Model file for the job. Use its own axes, mm. Face numbers are marked on the shaded views. Coordinates: 2 decimals unless noted, no trailing zeros. Order: outer loops, then holes, each group sorted by start corner. A loop starts at its lowest first (then second) coordinate and runs counter-clockwise, first axis right, second up. Notation, with made-up numbers: (-31.75, 49) -> (-9.75, 49) arc R24 cw to (-9.75, 65) -> close; hole circle Ø10 at (68.25, -12.75). An arc over 180 degrees is marked (long way). Write item = value, one per line. Start each with the question number.
Q1. Flat gauge pins, fed straight in: pin 1 (3 mm diameter, centred on x = 2.5, y = 112, fed in from +Z); pin 2 (7 mm diameter, centred on y = 99.36, z = 75.68, fed in from -X); pin 3 (4 mm diameter, centred on x = -19.05, z = -9.525, fed in from +Y); pin 4 (8 mm diameter, centred on x = -8, z = 86.5, fed in from +Y). Where does each tip first touch, or does it go through?
Q2. Cut at B-B, the plane y = 158.75. List the corners of the cut face in (x, z) (3 decimals), plus the area to 3 significant figures.
Q3. Cut at A-A, the plane x = -5. List the corners of the cut face in (y, z) (3 decimals).
Q4. Cut at D-D, the plane x = -23.5. List the corners of the cut face in (y, z) (3 decimals).
Q5. Cut at C-C, the plane y = 39. List the corners of the cut face in (x, z) (3 decimals).
Q6. Wall check: line 1 (Z direction, x = -19, y = 4) (3 decimals); line 2 (Y direction, x = -15.5, z = 73). Give the ranges that are in metal, low to high. Write a range as from..to.
Q7. Mould opens along Y. For the marked faces 1, 2 and 3 say: +Y half, -Y half, draft (parallel to the pull), parting line (faces both ways), or undercut.
from build123d import *

# Parameters (mm, degrees)
BOSS_EXTRUDE1_DEPTH  = 6.35
SKETCH5_W            = 184.15
SKETCH5_H            = 6.35
BOSS_EXTRUDE4_DEPTH  = 31.75
SKETCH6_W            = 12.7
SKETCH6_H            = 88.9
CUT_EXTRUDE2_DEPTH   = 270.576010849
CUT_EXTRUDE3_REACH   = 277.64
SKETCH7_R            = 2.25
SKETCH7_W            = 59.436
SKETCH7_H            = 28.313784743
SKETCH8_R            = 6.35
CUT_EXTRUDE4_DEPTH   = 276.640473489
FILLET1_R            = 2.54
CONVERT_SOLID1_START = -34.925
CONVERT_SOLID1_DEPTH = 184.15
CUT_EXTRUDE5_REACH   = 277.64
CUT_EXTRUDE6_REACH   = 271.576
SKETCH10_R           = 1.63195


# Read off the part's stored shape, not the designer's step: Convert-Solid1
with BuildPart() as part:
    # Sketch1 → Boss-Extrude1 (new body)
    with BuildSketch(Plane(origin=(0, 0, 0), x_dir=(0, 0, -1), z_dir=(1, 0, 0))):
        with BuildLine():
            Line((-117.475, 228.6), (34.925, 228.6))
            Line((34.925, 228.6), (34.925, 8.89))
            Line((34.925, 8.89), (34.925, 0))
            Line((34.925, 0), (-34.925, 0))
            Line((-34.925, 0), (-34.925, 8.89))
            ThreePointArc((-34.925, 8.89), (-79.375, 53.34), (-123.825, 8.89))
            Line((-123.825, 8.89), (-123.825, 0))
            Line((-123.825, 0), (-149.225, 0))
            Line((-149.225, 0), (-149.225, 76.2))
            Line((-149.225, 76.2), (-117.475, 228.6))
        make_face()
    extrude(amount=BOSS_EXTRUDE1_DEPTH)

    # Sketch5 → Boss-Extrude4 (add)
    with BuildSketch(Plane.ZY):
        with Locations((57.15, 3.175)):
            Rectangle(SKETCH5_W, SKETCH5_H)
    extrude(amount=BOSS_EXTRUDE4_DEPTH)

    # Sketch6 → Cut-Extrude2 (cut, through all)
    with BuildSketch(Plane(origin=(0, 6.35, 0), x_dir=(1, 0, 0), z_dir=(0, 1, 0))):
        with Locations((-6.35, -79.375)):
            Rectangle(SKETCH6_W, SKETCH6_H)
    extrude(amount=-CUT_EXTRUDE2_DEPTH, mode=Mode.SUBTRACT)

    # Sketch7 → Cut-Extrude3 (cut, up to next)
    with BuildSketch(Plane(origin=(6.35, 0, 0), x_dir=(0, 0, -1), z_dir=(1, 0, 0)), mode=Mode.PRIVATE) as cut_extrude3_sk1:
        with Locations((-75.679460058, 116.337237118)):
            Circle(SKETCH7_R)
    cut_extrude3_tool1 = extrude(cut_extrude3_sk1.sketch, amount=-CUT_EXTRUDE3_REACH, mode=Mode.PRIVATE) & part.part
    # Sketch7 → Cut-Extrude3 (cut, up to next)
    with BuildSketch(Plane(origin=(6.35, 0, 0), x_dir=(0, 0, -1), z_dir=(1, 0, 0)), mode=Mode.PRIVATE) as cut_extrude3_sk2:
        with Locations((-75.679460058, 99.360389657)):
            Circle(SKETCH7_R)
    cut_extrude3_tool2 = extrude(cut_extrude3_sk2.sketch, amount=-CUT_EXTRUDE3_REACH, mode=Mode.PRIVATE) & part.part
    # Sketch7 → Cut-Extrude3 (cut, up to next)
    with BuildSketch(Plane(origin=(6.35, 0, 0), x_dir=(0, 0, -1), z_dir=(1, 0, 0)), mode=Mode.PRIVATE) as cut_extrude3_sk3:
        with Locations((-6.03755368, 99.360389657)):
            Circle(SKETCH7_R)
    cut_extrude3_tool3 = extrude(cut_extrude3_sk3.sketch, amount=-CUT_EXTRUDE3_REACH, mode=Mode.PRIVATE) & part.part
    # Sketch7 → Cut-Extrude3 (cut, up to next)
    with BuildSketch(Plane(origin=(6.35, 0, 0), x_dir=(0, 0, -1), z_dir=(1, 0, 0)), mode=Mode.PRIVATE) as cut_extrude3_sk4:
        with Locations((-6.03755368, 116.337237118)):
            Circle(SKETCH7_R)
    cut_extrude3_tool4 = extrude(cut_extrude3_sk4.sketch, amount=-CUT_EXTRUDE3_REACH, mode=Mode.PRIVATE) & part.part
    # Sketch7 → Cut-Extrude3 (cut, up to next)
    with BuildSketch(Plane(origin=(6.35, 0, 0), x_dir=(0, 0, -1), z_dir=(1, 0, 0)), mode=Mode.PRIVATE) as cut_extrude3_sk5:
        with Locations((-40.858506869, 107.848813388)):
            Rectangle(SKETCH7_W, SKETCH7_H)
    cut_extrude3_tool5 = extrude(cut_extrude3_sk5.sketch, amount=-CUT_EXTRUDE3_REACH, mode=Mode.PRIVATE) & part.part
    add(cut_extrude3_tool1.solids().sort_by_distance((6.35, 116.337237, 75.67946))[0], mode=Mode.SUBTRACT)
    add(cut_extrude3_tool2.solids().sort_by_distance((6.35, 99.36039, 75.67946))[0], mode=Mode.SUBTRACT)
    add(cut_extrude3_tool3.solids().sort_by_distance((6.35, 99.36039, 6.037554))[0], mode=Mode.SUBTRACT)
    add(cut_extrude3_tool4.solids().sort_by_distance((6.35, 116.337237, 6.037554))[0], mode=Mode.SUBTRACT)
    add(cut_extrude3_tool5.solids().sort_by_distance((6.35, 107.848813, 40.858507))[0], mode=Mode.SUBTRACT)

    # Sketch8 → Cut-Extrude4 (cut, through all)
    with BuildSketch(Plane(origin=(6.35, 0, 0), x_dir=(0, 0, -1), z_dir=(1, 0, 0))):
        with Locations((-15.875, 209.55)):
            Circle(SKETCH8_R)
    extrude(amount=-CUT_EXTRUDE4_DEPTH, mode=Mode.SUBTRACT)

    # Fillet1
    fillet1_edges = [part.edges().sort_by_distance(p)[0] for p in [
        (0, 6.35, 136.525),
        (0, 6.35, 0),
    ]]
    fillet(fillet1_edges, radius=FILLET1_R)

    # Convert-Solid1 outline → Convert-Solid1 (cut)
    with BuildSketch(Plane.XY.offset(CONVERT_SOLID1_START)):
        with BuildLine():
            ThreePointArc((6.35, 8.89), (3.746179285, 2.603820715), (-2.54, 0))
            Line((-2.54, 0), (6.35, 0))
            Line((6.35, 0), (6.35, 8.89))
        make_face()
    extrude(amount=CONVERT_SOLID1_DEPTH, mode=Mode.SUBTRACT)

    # Sketch9 → Cut-Extrude5 (cut, up to next)
    with BuildSketch(Plane(origin=(6.35, 0, 0), x_dir=(0, 0, -1), z_dir=(1, 0, 0)), mode=Mode.PRIVATE) as cut_extrude5_sk1:
        with BuildLine():
            Line((-75.494212356, 184.752903033), (-73.141435562, 185.731480776))
            ThreePointArc((-73.141435562, 185.731480776), (-69.446832384, 185.812370314), (-66.675, 183.368279277))
            ThreePointArc((-66.675, 183.368279277), (-28.664883279, 153.84953873), (18.415, 163.83))
            ThreePointArc((18.415, 163.83), (27.305, 162.56), (26.035, 153.67))
            ThreePointArc((26.035, 153.67), (-31.616379009, 141.496848075), (-78.066338809, 177.749687467))
            ThreePointArc((-78.066338809, 177.749687467), (-78.311881244, 181.813820193), (-75.494212356, 184.752903033))
        make_face()
    cut_extrude5_tool1 = extrude(cut_extrude5_sk1.sketch, amount=-CUT_EXTRUDE5_REACH, mode=Mode.PRIVATE) & part.part
    # Sketch9 → Cut-Extrude5 (cut, up to next)
    with BuildSketch(Plane(origin=(6.35, 0, 0), x_dir=(0, 0, -1), z_dir=(1, 0, 0)), mode=Mode.PRIVATE) as cut_extrude5_sk2:
        with BuildLine():
            Line((-108.118493719, 66.728864942), (-90.609860799, 150.770302958))
            ThreePointArc((-90.609860799, 150.770302958), (-100.452693102, 165.793573316), (-115.47596346, 155.950741012))
            Line((-115.47596346, 155.950741012), (-132.98459638, 71.909302996))
            ThreePointArc((-132.98459638, 71.909302996), (-123.141764077, 56.886032638), (-108.118493719, 66.728864942))
        make_face()
    cut_extrude5_tool2 = extrude(cut_extrude5_sk2.sketch, amount=-CUT_EXTRUDE5_REACH, mode=Mode.PRIVATE) & part.part
    # Sketch9 → Cut-Extrude5 (cut, up to next)
    with BuildSketch(Plane(origin=(6.35, 0, 0), x_dir=(0, 0, -1), z_dir=(1, 0, 0)), mode=Mode.PRIVATE) as cut_extrude5_sk3:
        with BuildLine():
            Line((-40.087105739, 67.347842772), (1.2905656, 18.917236412))
            ThreePointArc((1.2905656, 18.917236412), (8.316769711, 17.084699632), (12.468452925, 23.041986075))
            Line((12.468452925, 23.041986075), (12.468863596, 71.472592434))
            ThreePointArc((12.468863596, 71.472592434), (10.609010694, 75.962755303), (6.118863596, 77.82264628))
            Line((6.118863596, 77.82264628), (-35.259218414, 77.82264628))
            ThreePointArc((-35.259218414, 77.82264628), (-41.026150106, 74.130652838), (-40.087105739, 67.347842772))
        make_face()
    cut_extrude5_tool3 = extrude(cut_extrude5_sk3.sketch, amount=-CUT_EXTRUDE5_REACH, mode=Mode.PRIVATE) & part.part
    # Sketch9 → Cut-Extrude5 (cut, up to next)
    with BuildSketch(Plane(origin=(6.35, 0, 0), x_dir=(0, 0, -1), z_dir=(1, 0, 0)), mode=Mode.PRIVATE) as cut_extrude5_sk4:
        with BuildLine():
            ThreePointArc((-61.255276679, 214.786351204), (-58.421011662, 192.917929262), (-45.672728213, 174.925091643))
            ThreePointArc((-45.672728213, 174.925091643), (-32.993270754, 175.875161813), (-33.943340924, 188.554619273))
            ThreePointArc((-33.943340924, 188.554619273), (-41.673471553, 199.464871288), (-43.392074603, 212.725147383))
            ThreePointArc((-43.392074603, 212.725147383), (-51.29307373, 222.687350332), (-61.255276679, 214.786351204))
        make_face()
    cut_extrude5_tool4 = extrude(cut_extrude5_sk4.sketch, amount=-CUT_EXTRUDE5_REACH, mode=Mode.PRIVATE) & part.part
    # Sketch9 → Cut-Extrude5 (cut, up to next)
    with BuildSketch(Plane(origin=(6.35, 0, 0), x_dir=(0, 0, -1), z_dir=(1, 0, 0)), mode=Mode.PRIVATE) as cut_extrude5_sk5:
        with BuildLine():
            ThreePointArc((-12.080418407, 164.026489196), (13.963017041, 174.959804504), (28.599113727, 199.117258578))
            ThreePointArc((28.599113727, 199.117258578), (21.899199613, 209.923850348), (11.092607844, 203.223936233))
            ThreePointArc((11.092607844, 203.223936233), (2.217770715, 188.575667985), (-13.574093253, 181.946073037))
            ThreePointArc((-13.574093253, 181.946073037), (-21.787047751, 172.239443693), (-12.080418407, 164.026489196))
        make_face()
    cut_extrude5_tool5 = extrude(cut_extrude5_sk5.sketch, amount=-CUT_EXTRUDE5_REACH, mode=Mode.PRIVATE) & part.part
    add(cut_extrude5_tool1.solids().sort_by_distance((6.35, 181.411079, 77.215324))[0], mode=Mode.SUBTRACT)
    add(cut_extrude5_tool2.solids().sort_by_distance((6.35, 111.339803, 111.797229))[0], mode=Mode.SUBTRACT)
    add(cut_extrude5_tool3.solids().sort_by_distance((6.35, 54.455432, 7.917782))[0], mode=Mode.SUBTRACT)
    add(cut_extrude5_tool4.solids().sort_by_distance((6.35, 197.006846, 47.961274))[0], mode=Mode.SUBTRACT)
    add(cut_extrude5_tool5.solids().sort_by_distance((6.35, 184.385964, -5.831872))[0], mode=Mode.SUBTRACT)

    # Sketch10 → Cut-Extrude6 (cut, up to next)
    with BuildSketch(Plane(origin=(0, 6.35, 0), x_dir=(1, 0, 0), z_dir=(0, 1, 0)), mode=Mode.PRIVATE) as cut_extrude6_sk1:
        with Locations(Location((-19.05, 9.525, 0), (0, 0, 270))):
            Circle(SKETCH10_R)
    cut_extrude6_tool1 = extrude(cut_extrude6_sk1.sketch, amount=-CUT_EXTRUDE6_REACH, mode=Mode.PRIVATE) & part.part
    # Sketch10 → Cut-Extrude6 (cut, up to next)
    with BuildSketch(Plane(origin=(0, 6.35, 0), x_dir=(1, 0, 0), z_dir=(0, 1, 0)), mode=Mode.PRIVATE) as cut_extrude6_sk2:
        with Locations(Location((-19.05, -15.875, 0), (0, 0, 270))):
            Circle(SKETCH10_R)
    cut_extrude6_tool2 = extrude(cut_extrude6_sk2.sketch, amount=-CUT_EXTRUDE6_REACH, mode=Mode.PRIVATE) & part.part
    # Sketch10 → Cut-Extrude6 (cut, up to next)
    with BuildSketch(Plane(origin=(0, 6.35, 0), x_dir=(1, 0, 0), z_dir=(0, 1, 0)), mode=Mode.PRIVATE) as cut_extrude6_sk3:
        with Locations(Location((-19.05, -142.875, 0), (0, 0, 270))):
            Circle(SKETCH10_R)
    cut_extrude6_tool3 = extrude(cut_extrude6_sk3.sketch, amount=-CUT_EXTRUDE6_REACH, mode=Mode.PRIVATE) & part.part
    add(cut_extrude6_tool1.solids().sort_by_distance((-19.05, 6.35, -9.525))[0], mode=Mode.SUBTRACT)
    add(cut_extrude6_tool2.solids().sort_by_distance((-19.05, 6.35, 15.875))[0], mode=Mode.SUBTRACT)
    add(cut_extrude6_tool3.solids().sort_by_distance((-19.05, 6.35, 142.875))[0], mode=Mode.SUBTRACT)


solid = part.part
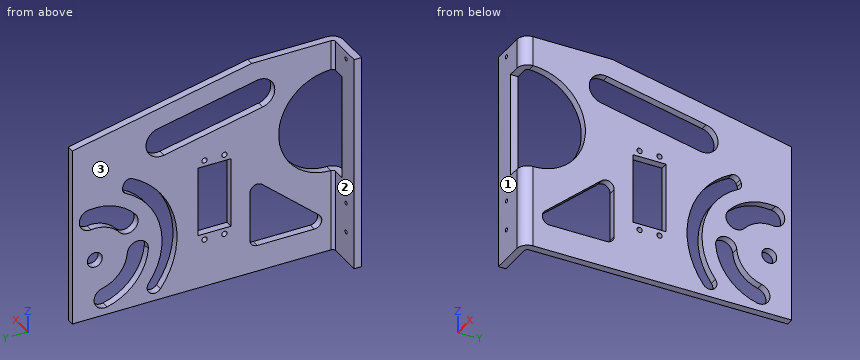
Here are the results:
q1.pin_1 = 142.08
q1.pin_2 = 0
q1.pin_3 = 6.35
q1.pin_4 = through
q2.outline = (0, -34.925) -> (6.35, -34.925) -> (6.35, -28.575) -> (0, -28.575) -> close; (0, -10.307) -> (6.35, -10.307) -> (6.35, 42.057) -> (0, 42.057) -> close; (0, 63.816) -> (6.35, 63.816) -> (6.35, 91.543) -> (0, 91.543) -> close; (0, 114.543) -> (6.35, 114.543) -> (6.35, 132.027) -> (0, 132.027) -> close
q2.area = 660 mm²
q3.outline = (0, -34.925) -> (6.35, -34.925) -> (6.35, 34.925) -> (0, 34.925) -> close; (0, 123.825) -> (6.35, 123.825) -> (6.35, 149.225) -> (0, 149.225) -> close
q4.outline = (0, -34.925) -> (6.35, -34.925) -> (6.35, 149.225) -> (0, 149.225) -> close
q5.outline = (0, -34.925) -> (6.35, -34.925) -> (6.35, -12.469) -> (0, -12.469) -> close; (0, 15.868) -> (6.35, 15.868) -> (6.35, 46.677) -> (0, 46.677) -> close; (0, 112.073) -> (6.35, 112.073) -> (6.35, 149.225) -> (0, 149.225) -> close
q6.line_1 = -34.925..-11.156, -7.894..14.244, 17.506..141.244, 144.506..149.225
q6.line_2 = 0..6.35
q7.face_1 = -Y half
q7.face_2 = +Y half
q7.face_3 = draft
